Design review of the part built by this model. Coordinates are the model's own, in mm. Round coordinates to 2 decimals unless told otherwise and drop trailing zeros. Write each loop counter-clockwise with the first axis right and the second up, starting at its lowest first coordinate (ties: lowest second). Pieces come first, ordered by that corner, then holes. Notation, with made-up numbers: M -32.75,36.25 L -20.75,36.25 A13 cw -20.75,54.25 Z; hole C 37,80.5 d4. An arc over 180 degrees is marked long. One line per question, with ' | ' between items. Start each with the question number.
Item 1: Add section A-A, the plane z = 0. State the section outline as (x, y) points.
Item 2: Add section C-C, the plane x = 63.5. State the section outline as (y, z) points.
Item 3: Add section B-B, the plane y = 4. State the section outline as (x, z) points.
Item 4: Add section D-D, the plane x = 8. State the section outline as (y, z) points.
Item 5: Insertion check: pin 1 Ø4 at (x, y) = (75, 3.5) entering from +Z; pin 2 Ø4 at (x, y) = (108, 2) entering from -Z; pin 3 Ø4 at (y, z) = (4.5, 7) entering from +X; pin 4 Ø5 at (x, z) = (0, 0) entering from -Y. Each pin has a flat end and moves straight along its axis. Give the tip position at first contact, or say it passes through.
Item 6: For L1, parallel to X at y = 3.5, z = 0; L2, parallel to X at y = 4.75, z = -2.75; L3, parallel to Z at x = 75, y = 5.25, list the stretches that pass through material, from the lowest coordinate up.
```python
from build123d import *

# Parameters (mm, degrees)
SKETCH_1_R      = 3
SKETCH_1_R_2    = 7
EXTRUDE_2_DEPTH = 8


with BuildPart() as part:
    # 草图1 → 凸台-拉伸2 (new body)
    with BuildSketch(Plane(origin=(0, 0, 0), x_dir=(1, 0, 0), z_dir=(0, 1, 0))):
        with BuildLine():
            ThreePointArc((0, 7), (-6.973362887, -0.610090199), (1.215537244, -6.893654271))
            Line((1.215537244, -6.893654271), (28.968829743, -2))
            Line((28.968829743, -2), (153.256910837, -2))
            Line((153.256910837, -2), (173.579798567, -9.396926208))
            ThreePointArc((173.579798567, -9.396926208), (186.914448614, -1.305261922), (176.128442573, 9.961946981))
            Line((176.128442573, 9.961946981), (142.273233663, 7))
            Line((142.273233663, 7), (0, 7))
        make_face()
        with Locations(Location((0, 0, 0), (0, 0, 270))):
            Circle(SKETCH_1_R, mode=Mode.SUBTRACT)
        with Locations(Location((177, 0, 0), (0, 0, 270))):
            Circle(SKETCH_1_R_2, mode=Mode.SUBTRACT)
    extrude(amount=EXTRUDE_2_DEPTH)


solid = part.part
```
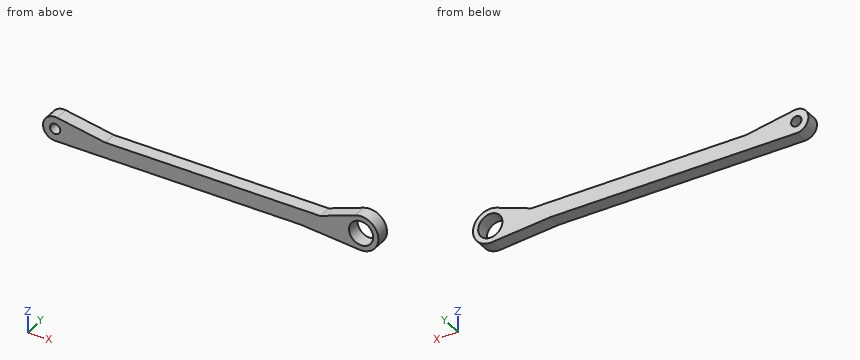
Computed values:
1) outline: M -7,0 L -3,0 L -3,8 L -7,8 Z; M 3,0 L 170,0 L 170,8 L 3,8 Z; M 184,0 L 187,0 L 187,8 L 184,8 Z
2) outline: M 0,-7 L 8,-7 L 8,2 L 0,2 Z
3) outline: M 0,-7 L 142.27,-7 L 176.13,-9.96 A10 ccw long 173.58,9.4 L 153.26,2 L 28.97,2 L 1.22,6.89 A7 ccw long Z; hole C 0,0 d6; hole C 177,0 d14
4) outline: M 0,-7 L 8,-7 L 8,5.7 L 0,5.7 Z
5) pin 1: stops at z = 2 | pin 2: stops at z = -7 | pin 3: stops at x = 185.66 | pin 4: passes through
6) L1: x = -7 to -3, 3 to 170, 184 to 187 | L2: x = -6.44 to -1.2, 1.2 to 170.56, 183.44 to 186.61 | L3: z = -7 to 2
